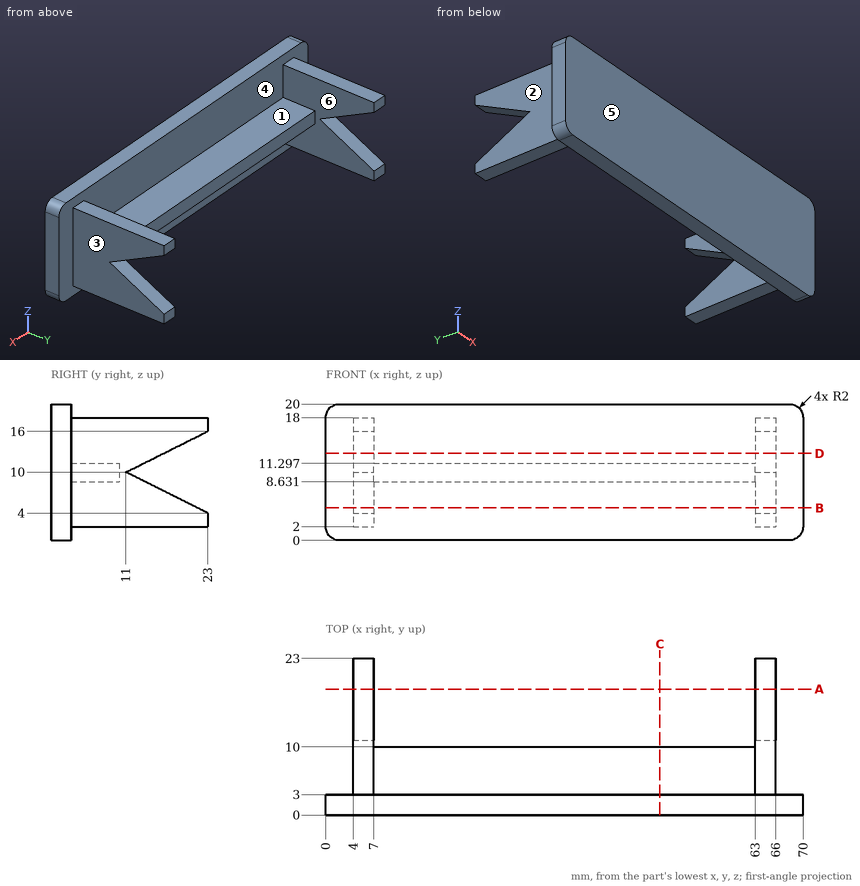
Check sheet for the drawn part. Datum: minimum x, y, z corner. Units: mm. A direction names the side the tool comes from. Coordinates: 2 decimals unless noted, no trailing zeros. Loops run counter-clockwise (first coordinate to the right, second up) from the corner with the lowest first, then second, coordinate; pieces in that order, holes last. Notation, with made-up numbers: (-3.75, -12) - (14.25, -12) arc R26 ccw to (14.25, 3) - close; hole circle Ø8 at (64.5, 7.25). An arc over 180 degrees is marked (long way). Put each result on its own line as item: value.
Item 1: Set-up check for the marked faces 5 and 6: record each of +Z, -Z, +X, -X, +Y, -Y from which the full face is reachable in a straight line by a thin tool's end or side.
Conclusion:
face 5: +Z, -Z, +X, -X, -Y
face 6: +Y
Item 2: Section check D-D (z = 12.75). Enter the section's corners in (x, y).
Conclusion:
outline: (0, 0) - (70, 0) - (70, 3) - (66, 3) - (66, 16.5) - (63, 16.5) - (63, 3) - (7, 3) - (7, 16.5) - (4, 16.5) - (4, 3) - (0, 3) - close
Item 3: Scan lines: line 1 along X through (y, z) = (5, 7); line 2 along Y through (x, z) = (61, 14.75); line 3 along Y through (x, z) = (13, 10.25). Record each from-to range of solid material in increasing order.
Conclusion:
line 1: x = 4 to 7, 63 to 66
line 2: y = 0 to 3
line 3: y = 0 to 10
Item 4: Section check B-B (z = 4.75). Enter the section's corners in (x, y).
Conclusion:
outline: (0, 0) - (70, 0) - (70, 3) - (66, 3) - (66, 21.5) - (63, 21.5) - (63, 3) - (7, 3) - (7, 21.5) - (4, 21.5) - (4, 3) - (0, 3) - close
Item 5: Gauge pin test, flat ends, axial feed: pin 1 Ø1.5 at (y, z) = (5, 15) entering from +X; pin 2 Ø1.5 at (x, y) = (64, 15.5) entering from -Z; pin 3 Ø1.5 at (y, z) = (6, 3) entering from -X. Record the tip position at first contact, or that the pin passes through.
Conclusion:
pin 1: stops at x = 66
pin 2: stops at z = 2
pin 3: stops at x = 4
Item 6: Section check C-C (x = 49). Enter the section's corners in (y, z).
Conclusion:
outline: (0, 0) - (3, 0) - (3, 8.63) - (10, 8.63) - (10, 11.3) - (3, 11.3) - (3, 20) - (0, 20) - close
Item 7: Section check A-A (y = 18.5). Enter the section's corners in (x, z).
Conclusion:
outline: (4, 2) - (7, 2) - (7, 6.25) - (4, 6.25) - close; (4, 13.75) - (7, 13.75) - (7, 18) - (4, 18) - close; (63, 2) - (66, 2) - (66, 6.25) - (63, 6.25) - close; (63, 13.75) - (66, 13.75) - (66, 18) - (63, 18) - close
Item 8: Draft check along X on the marked faces 1, 2, 3 and 4. Enter one of: pulls with the +X half, pulls with the -X half, needs draft (parallel to the pull), parting line crosses it, or undercut.
Conclusion:
face 1: undercut
face 2: pulls with the -X half
face 3: pulls with the +X half
face 4: undercut
